Part model, mm, in its own coordinate system. Face numbers are marked on the shaded views. Give positions to 0.01 mm unless a question says otherwise; leave off trailing zeros. Use a Markdown table: item, result. Add a question column.
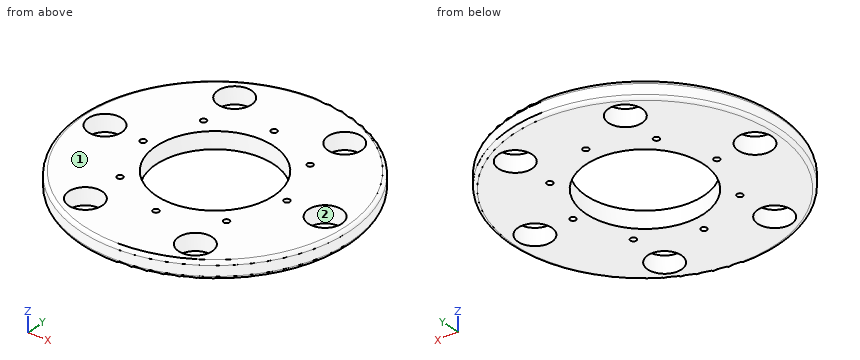
from build123d import *

# Parameters (mm, degrees)
SKETCH_3_R          = 80
EXTRUDE_1_DEPTH     = 10
SKETCH_4_R          = 35
CUT_EXTRUDE_1_DEPTH = 7
SKETCH_6_R          = 10
CUT_EXTRUDE_3_DEPTH = 10
SKETCH_5_R          = 1.75
CUT_EXTRUDE_4_DEPTH = 10
SKETCH_7_R          = 35
CUT_EXTRUDE_5_DEPTH = 20
FILLET_1_R          = 2


with BuildPart() as part:
    # 草图3 → 凸台-拉伸1 (new body)
    with BuildSketch(Plane.XY):
        Circle(SKETCH_3_R)
    extrude(amount=-EXTRUDE_1_DEPTH)

    # 草图4 → 切除-拉伸1 (cut)
    with BuildSketch(Plane.XY):
        Circle(SKETCH_4_R)
    extrude(amount=-CUT_EXTRUDE_1_DEPTH, mode=Mode.SUBTRACT)

    # 草图6 → 切除-拉伸3 (cut)
    with BuildSketch(Plane.XY):
        with Locations((-32.5, 56.291651246)):
            Circle(SKETCH_6_R)
        with BuildLine():
            ThreePointArc((-75, 0), (-65, -10), (-55, 0))
            Line((-55, 0), (-75, 0))
        make_face()
        with BuildLine():
            Line((-75, 0), (-55, 0))
            ThreePointArc((-55, 0), (-65, 10), (-75, 0))
        make_face()
        with Locations((-32.5, -56.291651246)):
            Circle(SKETCH_6_R)
        with Locations((32.5, -56.291651246)):
            Circle(SKETCH_6_R)
        with Locations((65, 0)):
            Circle(SKETCH_6_R)
        with Locations((32.5, 56.291651246)):
            Circle(SKETCH_6_R)
    extrude(amount=-CUT_EXTRUDE_3_DEPTH, mode=Mode.SUBTRACT)

    # 草图5 → 切除-拉伸4 (cut)
    with BuildSketch(Plane.XY):
        with Locations((0, 44.5)):
            Circle(SKETCH_5_R)
        with Locations((31.466251763, 31.466251763)):
            Circle(SKETCH_5_R)
        with Locations((42.5, 0)):
            Circle(SKETCH_5_R)
        with Locations((31.466251763, -31.466251763)):
            Circle(SKETCH_5_R)
        with Locations((-31.466251763, -31.466251763)):
            Circle(SKETCH_5_R)
        with BuildLine():
            ThreePointArc((-44.25, 0), (-42.5, -1.75), (-40.75, 0))
            Line((-40.75, 0), (-44.25, 0))
        make_face()
        with BuildLine():
            Line((-44.25, 0), (-40.75, 0))
            ThreePointArc((-40.75, 0), (-42.5, 1.75), (-44.25, 0))
        make_face()
        with Locations((-31.466251763, 31.466251763)):
            Circle(SKETCH_5_R)
        with Locations((0, -44.5)):
            Circle(SKETCH_5_R)
    extrude(amount=-CUT_EXTRUDE_4_DEPTH, mode=Mode.SUBTRACT)

    # 草图7 → 切除-拉伸5 (cut, symmetric)
    with BuildSketch(Plane.XY):
        Circle(SKETCH_7_R)
    extrude(amount=CUT_EXTRUDE_5_DEPTH, both=True, mode=Mode.SUBTRACT)

    # 圆角1
    fillet_1_edges = [part.edges().sort_by_distance(p)[0] for p in [
        (-80, 0, 0),
        (-80, 0, -10),
    ]]
    fillet(fillet_1_edges, radius=FILLET_1_R)


solid = part.part
1. Cut at A-A (z = -5.75). Give the number of separate pieces and of enclosed holes in the cut face, then the cut area to 3 significant figures.
2. Mould opens along X. For the marked faces 1 and 2 say: released by +X, released by -X, zero draft, split by the parting line, or undercut.
3. Flat gauge pins, fed straight in: pin 1 (3 mm diameter, centred on y = -21.5, z = -7.5, fed in from +X); pin 2 (1.5 mm diameter, centred on y = -32, z = -1.5, fed in from +X); pin 3 (1 mm diameter, centred on y = 55, z = -3.5, fed in from +X). Where does each tip first touch, or does it go through?
4. Drill centre lines: probe 1 along X at (y, z) = (52, -1); probe 2 along X at (y, z) = (-64.5, -7); probe 3 along Y at (x, z) = (-43, -9.5). Where is each one in solid material? Low to high. Write a range as [from, to].
A:
| question | item | result |
|---|---|---|
| 1 | separate pieces | 1 |
| 1 | enclosed holes | 15 |
| 1 | area | 14,300 mm² |
| 2 | face 1 | zero draft |
| 2 | face 2 | undercut |
| 3 | pin 1 | stops at x = 77.46 |
| 3 | pin 2 | stops at x = 73.61 |
| 3 | pin 3 | stops at x = 58.56 |
| 4 | probe 1 | x = [-60.44, -41.53], [-23.47, 23.47], [41.53, 60.44] |
| 4 | probe 2 | x = [-47.33, -38.21], [-26.79, 26.79], [38.21, 47.33] |
| 4 | probe 3 | y = [-66.66, -1.68], [1.68, 66.66] |
